Check sheet for the modelled part. Datum: model origin and axes. Units: mm. A direction names the side the tool comes from. Give positions to 0.01 mm unless a question says otherwise; leave off trailing zeros. Write each loop counter-clockwise with the first axis right and the second up, starting at its lowest first coordinate (ties: lowest second). Pieces come first, ordered by that corner, then holes. Notation, with made-up numbers: (60, 21) -> (96, 21) arc R24 cw to (96, 43) -> close; hole circle Ø4 at (-18, -16). An arc over 180 degrees is marked (long way). Return JSON: item names as keys, results as strings.
from build123d import *

# Parameters (mm, degrees)
SKETCH1_W           = 18.42
SKETCH1_H           = 18.42
BOSS_EXTRUDE1_DEPTH = 3.09
SKETCH2_W           = 16
SKETCH2_H           = 16
BOSS_EXTRUDE2_DEPTH = 2.5
SKETCH4_W           = 17
SKETCH4_H           = 17
CUT_EXTRUDE1_DEPTH  = 0.05


with BuildPart() as part:
    # Sketch1 → Boss-Extrude1 (new body)
    with BuildSketch(Plane(origin=(0, 0, 0), x_dir=(1, 0, 0), z_dir=(0, 1, 0))):
        Rectangle(SKETCH1_W, SKETCH1_H)
    extrude(amount=BOSS_EXTRUDE1_DEPTH)

    # Sketch2 → Boss-Extrude2 (add)
    with BuildSketch(Plane.XZ):
        Rectangle(SKETCH2_W, SKETCH2_H)
    extrude(amount=BOSS_EXTRUDE2_DEPTH)

    # Sketch4 → Cut-Extrude1 (cut)
    with BuildSketch(Plane(origin=(0, 3.09, 0), x_dir=(1, 0, 0), z_dir=(0, 1, 0))):
        Rectangle(SKETCH4_W, SKETCH4_H)
    extrude(amount=-CUT_EXTRUDE1_DEPTH, mode=Mode.SUBTRACT)


solid = part.part
(1) Cross-section at A-A on z = -4.5. Enter the section's corners in (x, y).
Reply:
{"outline": "(-9.21, 0) -> (-8, 0) -> (-8, -2.5) -> (8, -2.5) -> (8, 0) -> (9.21, 0) -> (9.21, 3.09) -> (8.5, 3.09) -> (8.5, 3.04) -> (-8.5, 3.04) -> (-8.5, 3.09) -> (-9.21, 3.09) -> close"}
(2) Depth check by flat-ended pin: pin 1 Ø1 at (x, y) = (-5, -1.5) entering from +Z; pin 2 Ø4 at (x, z) = (3.5, -2.5) entering from +Y; pin 3 Ø1.2 at (y, z) = (-1.5, -4) entering from +X. Enter the tip coordinate at first touch or a pass-through.
Reply:
{"pin 1": "z = 8", "pin 2": "y = 3.04", "pin 3": "x = 8"}
(3) Set-up check for faces 1 (the flat face through (0, -1, 8)), 2 (the flat face through (8, -1, 0)), 3 (the flat face through (0, -1, -8)): record each of +Z, -Z, +X, -X, +Y, -Y from which the full face is reachable in a straight line by a thin tool's end or side.
Reply:
{"face 1": "+Z, +X, -X, -Y", "face 2": "+Z, -Z, +X, -Y", "face 3": "-Z, +X, -X, -Y"}
(4) Thickness scan on L1, parallel to X at y = -1.4, z = -3.25; L2, parallel to Y at x = -7.5, z = 1.75. Record the ranges inside material, lowest first.
Reply:
{"L1": "-8 to 8", "L2": "-2.5 to 3.04"}
(5) Cross-section at B-B on x = 3. Enter the section's corners in (y, z).
Reply:
{"outline": "(-2.5, -8) -> (0, -8) -> (0, -9.21) -> (3.09, -9.21) -> (3.09, -8.5) -> (3.04, -8.5) -> (3.04, 8.5) -> (3.09, 8.5) -> (3.09, 9.21) -> (0, 9.21) -> (0, 8) -> (-2.5, 8) -> close"}
(6) Release check for a two-part mould opening along Z. For faces 4 (the flat face through (-9.21, 2, 0)), 5 (the flat face through (0, 2, 9.21)), 6 (the flat face through (0, 3.04, 0)), 7 (the flat face through (0, 2, -9.21)) record: pulls with the +Z half, pulls with the -Z half, needs draft (parallel to the pull), parting line crosses it, or undercut.
Reply:
{"face 4": "needs draft", "face 5": "pulls with the +Z half", "face 6": "undercut", "face 7": "pulls with the -Z half"}
